Geometry: final body of the model. Coordinates: model frame, mm. Face numbers are marked on the shaded views. A direction names the side the tool comes from. Give positions to 0.01 mm unless a question says otherwise; leave off trailing zeros. Write each loop counter-clockwise with the first axis right and the second up, starting at its lowest first coordinate (ties: lowest second). Pieces come first, ordered by that corner, then holes.
Q1. Section A-A (y = -87.5). Return the cut outline in (x, z).
Q2. Section B-B (x = 6). Return the cut outline in (y, z).
Q3. Mould query, pull axis X, two halves, no side actions, for the marked faces 1, 2, 3 and 4. Classes: +X half, -X half, draft (parallel to the pull), parting line (faces both ways), or undercut.
Q4. Line query: line 1 (X direction, y = -94, z = 226); line 2 (Z direction, x = 92, y = -9.5); line 3 (Z direction, x = -418.5, y = -43). Output: solid intervals per line, ascending.
Q5. Reachability of the marked faces 5, 6 and 7 from +Z, -Z, +X, -X, +Y, -Y: full face, straight path, thin tool, end or side. Return the list, or none.
Q6. Section C-C (z = 111). Return the cut outline in (x, y).
Q7. Pin query (flat end, axial travel): pin 1 Ø2 at (x, y) = (-57.5, -76) entering from +Z; pin 2 Ø12.5 at (x, z) = (254, -269.5) entering from -Y. Return the tip coordinate at first contact, or that it passes through.
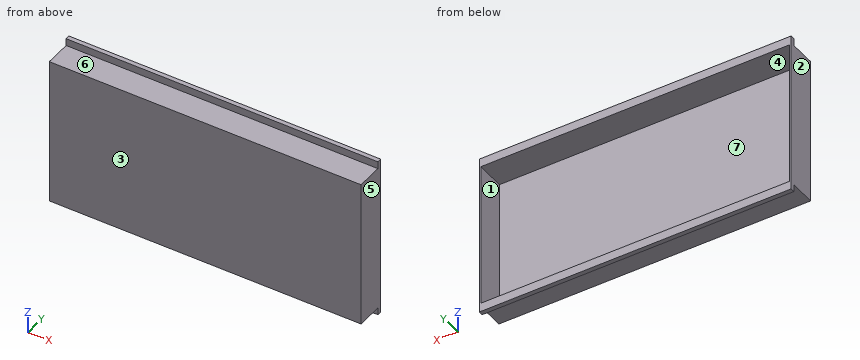
from build123d import *

# Parameters (mm, degrees)
CROQUIS1_W            = 1070
CROQUIS1_H            = 510
CROQUIS1_W_2          = 1060
CROQUIS1_H_2          = 500
EXTRUIR_L_MINA1_DEPTH = 100
CROQUIS2_W            = 1070
CROQUIS2_H            = 510
EXTRUIR1_DEPTH        = 5
CROQUIS3_W            = 1070
CROQUIS3_H            = 25
EXTRUIR2_DEPTH        = 15


with BuildPart() as part:
    # Croquis1 → Extruir-Lámina1 (new body)
    with BuildSketch(Plane(origin=(0, 0, 0), x_dir=(1, 0, 0), z_dir=(0, 1, 0))):
        Rectangle(CROQUIS1_W, CROQUIS1_H)
        Rectangle(CROQUIS1_W_2, CROQUIS1_H_2, mode=Mode.SUBTRACT)
    extrude(amount=-EXTRUIR_L_MINA1_DEPTH)

    # Croquis2 → Extruir1 (add)
    with BuildSketch(Plane.XZ.offset(100)):
        Rectangle(CROQUIS2_W, CROQUIS2_H)
    extrude(amount=EXTRUIR1_DEPTH)

    # Croquis3 → Extruir2 (add)
    with BuildSketch(Plane(origin=(0, 0, 0), x_dir=(1, 0, 0), z_dir=(0, 1, 0))):
        with Locations((0, 267.5)):
            Rectangle(CROQUIS3_W, CROQUIS3_H)
        with Locations((0, -267.5)):
            Rectangle(CROQUIS3_W, CROQUIS3_H)
    extrude(amount=-EXTRUIR2_DEPTH)


solid = part.part
Computed:
1. outline: (-535, -255) - (535, -255) - (535, 255) - (-535, 255) - close; hole (-530, -250) - (530, -250) - (530, 250) - (-530, 250) - close
2. outline: (-105, -255) - (-15, -255) - (-15, -280) - (0, -280) - (0, -250) - (-100, -250) - (-100, 250) - (0, 250) - (0, 280) - (-15, 280) - (-15, 255) - (-105, 255) - close
3. face 1: undercut
3. face 2: -X half
3. face 3: draft
3. face 4: undercut
4. line 1: x = -535 to -530, 530 to 535
4. line 2: z = -280 to -250, 250 to 280
4. line 3: z = -255 to -250, 250 to 255
5. face 5: +Z, -Z, +X, +Y, -Y
5. face 6: +Z, +X, -X, -Y
5. face 7: +Y
6. outline: (-535, -105) - (535, -105) - (535, 0) - (530, 0) - (530, -100) - (-530, -100) - (-530, 0) - (-535, 0) - close
7. pin 1: stops at z = 255
7. pin 2: stops at y = -15
